For this review, take the finished solid that the model builds, in its own axes (mm). A direction names the side the tool comes from. Round coordinates to 2 decimals unless told otherwise and drop trailing zeros. Loops run counter-clockwise (first coordinate to the right, second up) from the corner with the lowest first, then second, coordinate; pieces in that order, holes last.
1) Take a section at D-D (z = 16). State the section outline as (x, y) points.
2) Take a section at A-A (y = 2.5). State the section outline as (x, z) points, then the cut area to 3 significant figures.
3) Mouldability with a two-part tool opening along X and no side actions: class faces 1 (the flat face through (-22, 2, -22)), 2 (the flat face through (22, 2, -22)), 3 (the cylindrical face through (-20.51, 2.22, -20.61)) as pulls with the +X half, pulls with the -X half, needs draft (parallel to the pull), parting line crosses it, or undercut.
4) Wall thickness on L1, parallel to X at y = 4.15, z = 0; L2, parallel to X at y = 3.4, z = 2; L3, parallel to X at y = 2.8, z = 0: over which ranges is each line inside the solid? List them lowest first.
5) Tool access review of faces 4 (the flat face through (8.4, 4.5, -8.9)), 5 (the flat face through (-17.4, 3.3, 9.5)): name each direction out of +Z, -Z, +X, -X, +Y, -Y from which nothing blocks a thin tool from reaching the whole face with its end or side.
6) Take a section at C-C (z = -5.5). State the section outline as (x, y) points, then the cut area to 3 significant figures.
7) Take a section at B-B (x = 0). State the section outline as (y, z) points.
```python
from build123d import *

# Parameters (mm, degrees)
SKETCH_1_W          = 45
SKETCH_1_H          = 45
EXTRUDE_1_DEPTH     = 4.5
SKETCH_2_R          = 5.5
CUT_EXTRUDE_1_DEPTH = 3.5
SKETCH_3_R          = 4
CUT_EXTRUDE_2_DEPTH = 33.011716605
SKETCH_4_R          = 12
SKETCH_4_R_2        = 9.5
CUT_EXTRUDE_3_DEPTH = 3
SKETCH_5_R          = 21.5
SKETCH_5_R_2        = 19.5
CUT_EXTRUDE_4_DEPTH = 1.2
CHAMFER_1_SIZE      = 1
SKETCH_6_R          = 1.5
CUT_EXTRUDE_5_DEPTH = 33.136427928


with BuildPart() as part:
    # 草图1 → 凸台-拉伸1 (new body)
    with BuildSketch(Plane(origin=(0, 0, 0), x_dir=(1, 0, 0), z_dir=(0, 1, 0))):
        Rectangle(SKETCH_1_W, SKETCH_1_H)
    extrude(amount=EXTRUDE_1_DEPTH)

    # 草图2 → 切除-拉伸1 (cut)
    with BuildSketch(Plane(origin=(0, 4.5, 0), x_dir=(1, 0, 0), z_dir=(0, 1, 0))):
        with Locations(Location((0, 3, 0), (0, 0, 270))):
            Circle(SKETCH_2_R)
    extrude(amount=-CUT_EXTRUDE_1_DEPTH, mode=Mode.SUBTRACT)

    # 草图3 → 切除-拉伸2 (cut, through all)
    with BuildSketch(Plane(origin=(0, 1, 0), x_dir=(1, 0, 0), z_dir=(0, 1, 0))):
        with Locations(Location((0, 3, 0), (0, 0, 270))):
            Circle(SKETCH_3_R)
    extrude(amount=-CUT_EXTRUDE_2_DEPTH, mode=Mode.SUBTRACT)

    # 草图4 → 切除-拉伸3 (cut)
    with BuildSketch(Plane(origin=(0, 4.5, 0), x_dir=(1, 0, 0), z_dir=(0, 1, 0))):
        with Locations(Location((0, 0, 0), (0, 0, 270))):
            Circle(SKETCH_4_R)
        with Locations(Location((0, 0, 0), (0, 0, 270))):
            Circle(SKETCH_4_R_2, mode=Mode.SUBTRACT)
    extrude(amount=-CUT_EXTRUDE_3_DEPTH, mode=Mode.SUBTRACT)

    # 草图5 → 切除-拉伸4 (cut)
    with BuildSketch(Plane(origin=(0, 4.5, 0), x_dir=(1, 0, 0), z_dir=(0, 1, 0))):
        with Locations(Location((0, 0, 0), (0, 0, 270))):
            Circle(SKETCH_5_R)
        with Locations(Location((0, 0, 0), (0, 0, 270))):
            Circle(SKETCH_5_R_2, mode=Mode.SUBTRACT)
    extrude(amount=-CUT_EXTRUDE_4_DEPTH, mode=Mode.SUBTRACT)

    # 倒角1
    chamfer_1_edges = [part.edges().sort_by_distance(p)[0] for p in [
        (22.5, 2.25, 22.5),
        (-22.5, 2.25, 22.5),
        (-22.5, 2.25, -22.5),
        (22.5, 2.25, -22.5),
    ]]
    chamfer(chamfer_1_edges, length=CHAMFER_1_SIZE)

    # 草图6 → 切除-拉伸5 (cut, through all)
    with BuildSketch(Plane.XZ):
        with Locations(Location((-19.5, 19.5, 0), (0, 0, 270))):
            Circle(SKETCH_6_R)
        with Locations(Location((19.5, 19.5, 0), (0, 0, 90))):
            Circle(SKETCH_6_R)
        with Locations(Location((19.5, -19.5, 0), (0, 0, 270))):
            Circle(SKETCH_6_R)
        with Locations(Location((-19.5, -19.5, 0), (0, 0, 90))):
            Circle(SKETCH_6_R)
    extrude(amount=-CUT_EXTRUDE_5_DEPTH, mode=Mode.SUBTRACT)


solid = part.part
```
Response:
1. outline: (-22.5, 0) - (22.5, 0) - (22.5, 4.5) - (14.36, 4.5) - (14.36, 3.3) - (11.15, 3.3) - (11.15, 4.5) - (-11.15, 4.5) - (-11.15, 3.3) - (-14.36, 3.3) - (-14.36, 4.5) - (-22.5, 4.5) - close
2. outline: (-22.5, -21.5) - (-21.5, -22.5) - (21.5, -22.5) - (22.5, -21.5) - (22.5, 21.5) - (21.5, 22.5) - (-21.5, 22.5) - (-22.5, 21.5) - close; circle Ø19 at (0, 0); hole circle Ø3 at (-19.5, -19.5); hole circle Ø3 at (-19.5, 19.5); hole circle Ø24 at (0, 0); hole circle Ø11 at (0, -3); hole circle Ø3 at (19.5, -19.5); hole circle Ø3 at (19.5, 19.5)
2. area: 1,730 mm2
3. face 1: pulls with the -X half
3. face 2: pulls with the +X half
3. face 3: undercut
4. L1: x = -22.5 to -21.5, -19.5 to -12, -9.5 to -4.61, 4.61 to 9.5, 12 to 19.5, 21.5 to 22.5
4. L2: x = -22.5 to -21.41, -19.4 to -11.83, -9.29 to -2.29, 2.29 to 9.29, 11.83 to 19.4, 21.41 to 22.5
4. L3: x = -22.5 to -12, -9.5 to -4.61, 4.61 to 9.5, 12 to 22.5
5. face 4: +Z, -Z, +X, -X, +Y
5. face 5: +Y
6. outline: (-22.5, 0) - (-3.12, 0) - (-3.12, 1) - (-4.9, 1) - (-4.9, 4.5) - (-7.75, 4.5) - (-7.75, 1.5) - (-10.67, 1.5) - (-10.67, 4.5) - (-18.71, 4.5) - (-18.71, 3.3) - (-20.78, 3.3) - (-20.78, 4.5) - (-22.5, 4.5) - close; (3.12, 0) - (22.5, 0) - (22.5, 4.5) - (20.78, 4.5) - (20.78, 3.3) - (18.71, 3.3) - (18.71, 4.5) - (10.67, 4.5) - (10.67, 1.5) - (7.75, 1.5) - (7.75, 4.5) - (4.9, 4.5) - (4.9, 1) - (3.12, 1) - close
6. area: 139 mm2
7. outline: (0, -22.5) - (4.5, -22.5) - (4.5, -21.5) - (3.3, -21.5) - (3.3, -19.5) - (4.5, -19.5) - (4.5, -12) - (1.5, -12) - (1.5, -9.5) - (4.5, -9.5) - (4.5, -8.5) - (1, -8.5) - (1, -7) - (0, -7) - close; (0, 1) - (1, 1) - (1, 2.5) - (4.5, 2.5) - (4.5, 9.5) - (1.5, 9.5) - (1.5, 12) - (4.5, 12) - (4.5, 19.5) - (3.3, 19.5) - (3.3, 21.5) - (4.5, 21.5) - (4.5, 22.5) - (0, 22.5) - close
